Geometry check sheet. Reference: the model listing, model coordinates, mm. Face numbers are marked on the shaded views. A direction names the side the tool comes from. Give positions to 0.01 mm unless a question says otherwise; leave off trailing zeros. Loops run counter-clockwise (first coordinate to the right, second up) from the corner with the lowest first, then second, coordinate; pieces in that order, holes last. Notation, with made-up numbers: (58, -33) -> (66, -33) arc R23 cw to (66, -21) -> close; hole circle Ø2 at (29, 50.25). An arc over 180 degrees is marked (long way). One line per item, written item: value. Start each with the question number.
(1) Sectioned sample at D-D, the plane z = -10. State how many separate pieces and enclosed holes the cut face has, then the cut area to 3 significant figures.
(2) Sectioned sample at A-A, the plane y = 25. Record the cut outline in (x, z).
(3) Sectioned sample at B-B, the plane z = 25.5. Record the cut outline in (x, y).
(4) Tool access check on the marked faces 1, 2 and 3. Record the directions out of +Z, -Z, +X, -X, +Y, -Y that give a thin tool (end or side, any length) a straight path to the whole face; none if there is none.
(5) Draft check along Z on the marked faces 4, 5 and 6. Enter one of: pulls with the +Z half, pulls with the -Z half, needs draft (parallel to the pull), parting line crosses it, or undercut.
(6) Scan lines: line 1 along Z through (x, y) = (66, -11.5); line 2 along X through (y, z) = (57, -9); line 3 along Z through (x, y) = (20.5, 31.5). Record each from-to range of solid material in increasing order. Write a range as from..to.
(7) Gauge pin test, flat ends, axial feed: pin 1 Ø6 at (x, y) = (13, 46) entering from +Z; pin 2 Ø4 at (y, z) = (25, -10) entering from +X; pin 3 Ø8 at (x, z) = (15, -6) entering from -Y; pin 4 Ø6 at (x, y) = (20.5, 10) entering from -Z. Record the tip position at first contact, or that the pin passes through.
(8) Sectioned sample at C-C, the plane x = 73. Record the cut outline in (y, z), then the cut area to 3 significant figures.
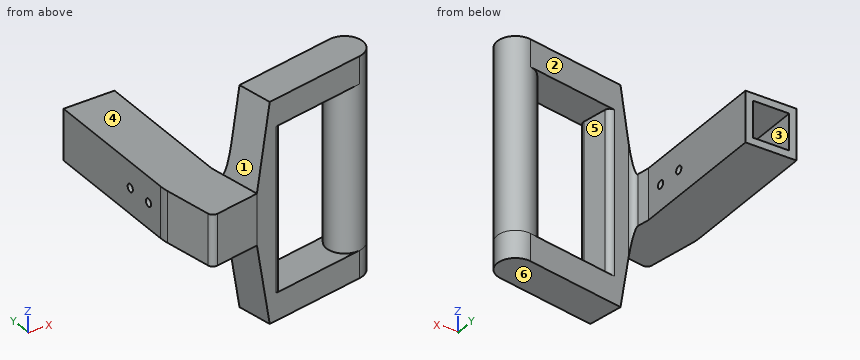
from build123d import *

# Parameters (mm, degrees)
SKETCH1_W                       = 28
SKETCH1_H                       = 28
SKETCH1_W_2                     = 20
SKETCH1_H_2                     = 20
BOSS_EXTRUDE1_DEPTH             = 30
SKETCH2_W                       = 28
SKETCH2_H                       = 28
BOSS_EXTRUDE2_DEPTH             = 3
SKETCH3_R                       = 2.15
CUT_EXTRUDE1_DEPTH              = 48.539457296
BOSS_EXTRUDE3_DEPTH             = 28
BOSS_EXTRUDE4_DEPTH             = 20
BOSS_EXTRUDE5_REACH             = 146.565
SKETCH6_R                       = 10
BOSS_EXTRUDE5_DIRECTION_2_REACH = 146.565
SKETCH7_W                       = 28
SKETCH7_H                       = 28
SKETCH7_W_2                     = 20
SKETCH7_H_2                     = 20
BOSS_EXTRUDE6_DEPTH             = 50
FILLET1_R                       = 3


with BuildPart() as part:
    # Sketch1 → Boss-Extrude1 (new body)
    with BuildSketch(Plane(origin=(0, 0, 0), x_dir=(1, 0, 0), z_dir=(0, 1, 0))):
        with Locations((10, 10)):
            Rectangle(SKETCH1_W, SKETCH1_H)
        with Locations((10, 10)):
            Rectangle(SKETCH1_W_2, SKETCH1_H_2, mode=Mode.SUBTRACT)
    extrude(amount=BOSS_EXTRUDE1_DEPTH)

    # Sketch2 → Boss-Extrude2 (add)
    with BuildSketch(Plane.XZ):
        with Locations((10, -10)):
            Rectangle(SKETCH2_W, SKETCH2_H)
    extrude(amount=-BOSS_EXTRUDE2_DEPTH)

    # Sketch3 → Cut-Extrude1 (cut, through all)
    with BuildSketch(Plane(origin=(24, 0, 0), x_dir=(0, 0, -1), z_dir=(1, 0, 0))):
        with Locations((10, 25)):
            Circle(SKETCH3_R)
        with Locations((10, 10)):
            Circle(SKETCH3_R)
    extrude(amount=-CUT_EXTRUDE1_DEPTH, mode=Mode.SUBTRACT)

    # Sketch4 → Boss-Extrude3 (add)
    with BuildSketch(Plane.XY.offset(4)):
        with BuildLine():
            Line((24, 0), (29.20944533, -29.54423259))
            Line((29.20944533, -29.54423259), (1.634828246, -34.406381565))
            Line((1.634828246, -34.406381565), (-3.574617084, -4.862148975))
            ThreePointArc((-3.574617084, -4.862148975), (-3.893451547, -2.440360797), (-4, 0))
            Line((-4, 0), (24, 0))
        make_face()
    extrude(amount=-BOSS_EXTRUDE3_DEPTH)

    # Sketch5 → Boss-Extrude4 (add)
    with BuildSketch(Plane(origin=(5.933133881, -33.64847431, 0), x_dir=(0, 0, -1), z_dir=(0.1736481776669318, -0.9848077530122078, 0))):
        Polygon((24, 23.635386072), (-4, 23.635386072), (-50, 31.746427185), (-50, 88.635386072), (-35, 88.635386072), (-35, 38.635386072), (55, 38.635386072), (55, 88.635386072), (70, 88.635386072), (70, 31.746427185), align=None)
    extrude(amount=-BOSS_EXTRUDE4_DEPTH)

    # Boss-Extrude5: up to this face of the body (flat: up to its plane)
    boss_extrude5_end = Plane(part.part.faces().sort_by_distance((63.473123613, -13.348355532, 50))[0])
    # Sketch6 → Boss-Extrude5 (add, up to the picked face)
    with BuildSketch(Plane.XY.offset(-55), mode=Mode.PRIVATE) as boss_extrude5_sk1:
        with Locations(Location((91.485467499, -8.409023512, 0), (0, 0, 100))):
            Circle(SKETCH6_R)
    boss_extrude5_tool1 = split(extrude(boss_extrude5_sk1.sketch, amount=BOSS_EXTRUDE5_REACH, mode=Mode.PRIVATE), bisect_by=boss_extrude5_end, keep=Keep.BOTH, mode=Mode.PRIVATE)
    add(boss_extrude5_tool1.solids().sort_by(Axis((91.485467, -8.409024, -55), (0, 0, 1)))[0])

    # Boss-Extrude5 direction 2: up to this face of the body (flat: up to its plane)
    boss_extrude5_direction_2_end = Plane(part.part.faces().sort_by_distance((63.473123613, -13.348355532, -70))[0])
    # Sketch6 → Boss-Extrude5 direction 2 (add, up to the picked face)
    with BuildSketch(Plane.XY.offset(-55), mode=Mode.PRIVATE) as boss_extrude5_direction_2_sk1:
        with Locations(Location((91.485467499, -8.409023512, 0), (0, 0, 100))):
            Circle(SKETCH6_R)
    boss_extrude5_direction_2_tool1 = split(extrude(boss_extrude5_direction_2_sk1.sketch, amount=-BOSS_EXTRUDE5_DIRECTION_2_REACH, mode=Mode.PRIVATE), bisect_by=boss_extrude5_direction_2_end, keep=Keep.BOTH, mode=Mode.PRIVATE)
    add(boss_extrude5_direction_2_tool1.solids().sort_by(Axis((91.485467, -8.409024, -55), (0, 0, -1)))[0])

    # Sketch7 → Boss-Extrude6 (add)
    with BuildSketch(Plane(origin=(0, 30, 0), x_dir=(1, 0, 0), z_dir=(0, 1, 0))):
        with Locations((10, 10)):
            Rectangle(SKETCH7_W, SKETCH7_H)
        with Locations((10, 10)):
            Rectangle(SKETCH7_W_2, SKETCH7_H_2, mode=Mode.SUBTRACT)
    extrude(amount=BOSS_EXTRUDE6_DEPTH)

    # Fillet1
    fillet1_edges = [part.edges().sort_by_distance(p)[0] for p in [
        (1.634828246, -34.406381565, -10),
        (25.736481777, -9.84807753, -10),
        (40.508598072, -7.243354865, -10),
        (43.981561625, -26.939509925, -10),
    ]]
    fillet(fillet1_edges, radius=FILLET1_R)


solid = part.part
Calculated:
1. separate pieces: 6
1. enclosed holes: 0
1. area: 2,150 mm2
2. outline: (-4, -24) -> (24, -24) -> (24, -12.15) -> (20, -12.15) -> (20, -20) -> (0, -20) -> (0, -12.15) -> (-4, -12.15) -> close; (-4, -7.85) -> (0, -7.85) -> (0, 0) -> (20, 0) -> (20, -7.85) -> (24, -7.85) -> (24, 4) -> (-4, 4) -> close
3. outline: (29.47, -9.19) -> (32.94, -28.89) -> (41.03, -27.46) arc R3 ccw to (43.46, -23.99) -> (41.03, -10.2) arc R3 ccw to (37.55, -7.76) -> close; circle Ø20 at (91.49, -8.41)
4. face 1: +Z, -X, -Y
4. face 2: +Z, -Z, +Y
4. face 3: +Y
5. face 4: pulls with the +Z half
5. face 5: undercut
5. face 6: pulls with the -Z half
6. line 1: z = -70..-55, 35..50
6. line 2: x = -4..0, 20..24
6. line 3: z = -24..4
7. pin 1: stops at z = 4
7. pin 2: passes through
7. pin 3: stops at y = -32.76
7. pin 4: stops at z = -24
8. outline: (-21.82, -70) -> (-1.51, -70) -> (-1.51, -55) -> (-21.82, -55) -> close; (-21.82, 35) -> (-1.51, 35) -> (-1.51, 50) -> (-21.82, 50) -> close
8. area: 609 mm2
